```python
from build123d import *

# Parameters (mm, degrees)
CROQUIS1_R              = 10
SALIENTE_EXTRUIR1_DEPTH = 100
CROQUIS2_R              = 7.5
SALIENTE_EXTRUIR2_DEPTH = 15
CROQUIS3_R              = 5
SALIENTE_EXTRUIR3_DEPTH = 16
REDONDEO1_R             = 4
CHAFL_N1_SIZE           = 1.99
CHAFL_N1_SIZE2          = 0.496162726
CROQUIS4_W              = 3.793672416
CROQUIS4_H              = 8.169837842
SALIENTE_EXTRUIR4_DEPTH = 16
CHAFL_N2_SIZE           = 12
CHAFL_N2_SIZE2          = 6.38051318
REDONDEO2_R             = 10


with BuildPart() as part:
    # Croquis1 → Saliente-Extruir1 (new body)
    with BuildSketch(Plane(origin=(0, 0, 0), x_dir=(1, 0, 0), z_dir=(0, 1, 0))):
        with Locations(Location((0, 0, 0), (0, 0, 270))):
            Circle(CROQUIS1_R)
    extrude(amount=SALIENTE_EXTRUIR1_DEPTH)

    # Croquis2 → Saliente-Extruir2 (add)
    with BuildSketch(Plane.XZ):
        with Locations(Location((0, 0, 0), (0, 0, 270))):
            Circle(CROQUIS2_R)
    extrude(amount=SALIENTE_EXTRUIR2_DEPTH)

    # Croquis3 → Saliente-Extruir3 (add)
    with BuildSketch(Plane.XZ.offset(15)):
        with Locations(Location((0, 0, 0), (0, 0, 270))):
            Circle(CROQUIS3_R)
    extrude(amount=SALIENTE_EXTRUIR3_DEPTH)

    # Redondeo1
    # the kernel refuses this fillet: 4 mm, written as the material it takes off along each edge
    with BuildSketch(Plane(origin=(0, 0, 0), x_dir=(0, 0, 1), z_dir=(-1, 0, 0))) as redondeo1_piece_1:
        with BuildLine():
            CenterArc((6, 3.708099244), REDONDEO1_R, 292.024312837, 67.975687163)
            Line((7.5, 0), (7.53, -0.074161985))
            ThreePointArc((7.53, -0.074161985), (8.75, -0.08), (10, -0.08))
            Line((10, -0.08), (10.08, 0))
            Line((10.08, 0), (10.08, 3.708099244))
            Line((10.08, 3.708099244), (10, 3.708099244))
        make_face()
    revolve(axis=Axis((0, 0, 0), (0, 1, 0)), mode=Mode.SUBTRACT)

    # Chaflán1
    chafl_n1_edges = [part.edges().sort_by_distance(p)[0] for p in [
        (0, -31, 5),
    ]]
    chafl_n1_side = [part.faces().sort_by_distance(p)[0] for p in [
        (0, -23, 5),
    ]]
    chamfer(chafl_n1_edges, length=CHAFL_N1_SIZE, length2=CHAFL_N1_SIZE2, reference=chafl_n1_side[0])

    # Croquis4 → Saliente-Extruir4 (add)
    with BuildSketch(Plane.XZ.offset(31)):
        Rectangle(CROQUIS4_W, CROQUIS4_H)
    extrude(amount=SALIENTE_EXTRUIR4_DEPTH)

    # Chaflán2
    chafl_n2_edges = [part.edges().sort_by_distance(p)[0] for p in [
        (0, -47, -4.084918921),
    ]]
    chafl_n2_side = [part.faces().sort_by_distance(p)[0] for p in [
        (0, -39, -4.084918921),
    ]]
    chamfer(chafl_n2_edges, length=CHAFL_N2_SIZE, length2=CHAFL_N2_SIZE2, reference=chafl_n2_side[0])

    # Redondeo2
    redondeo2_edges = [part.edges().sort_by_distance(p)[0] for p in [
        (0, 100, -10),
    ]]
    fillet(redondeo2_edges, radius=REDONDEO2_R)


solid = part.part
```
The model under review builds one solid part; all positions refer to its coordinate system, in mm. A direction names the side the tool comes from. Give positions to 0.01 mm unless a question says otherwise; leave off trailing zeros. Write each loop counter-clockwise with the first axis right and the second up, starting at its lowest first coordinate (ties: lowest second). Pieces come first, ordered by that corner, then holes. Notation, with made-up numbers: M 9,87.25 L 21,87.25 A21 ccw 21,96.25 Z; hole C 58.5,20.25 d3. An arc over 180 degrees is marked long. Answer in a Markdown table with one row per item.
Item 1: Tool access review of faces 1 (the face through (0, -39, 4.085)), 2 (the face through (0, -33, -4.085)), 3 (the face through (-3, -31, 0)), 4 (the face through (-4.88, -21.91, 1.08)): name each direction out of +Z, -Z, +X, -X, +Y, -Y from which nothing blocks a thin tool from reaching the whole face with its end or side.
Check sheet entries:
| item | result |
|---|---|
| face 1 | +Z, +X, -X, -Y |
| face 2 | -Z, +X, -X, -Y |
| face 3 | +Z, -Z, -X, -Y |
| face 4 | -Y |
Item 2: Add section A-A on x = 0. Give the boundary of the cut face in (y, z).
Check sheet entries:
| item | result |
|---|---|
| outline | M -47,2.3 L -35,-4.08 L -31,-4.08 L -31,-4.5 L -29.01,-5 L -15,-5 L -15,-7.5 L 0,-7.5 A4 ccw 3.71,-10 L 90,-10 A10 ccw 90,10 L 3.71,10 A4 ccw 0,7.5 L -15,7.5 L -15,5 L -29.01,5 L -31,4.5 L -31,4.08 L -47,4.08 Z |
Item 3: Add section C-C on y = -19. Give the boundary of the cut face in (x, z), plus the area to 3 significant figures.
Check sheet entries:
| item | result |
|---|---|
| outline | C 0,0 d10 |
| area | 78.5 mm2 |
Item 4: For P1, Ø8, axis at x = 2.5, z = -8, coming from the -Y side; P2, Ø10, axis at x = 7.5, y = 32.5, coming from the -Z side; P3, Ø2, axis at x = -5, z = -6, coming from the -Y side, all flat-tipped, find the tip position at first contact; note any pin that passes through.
Check sheet entries:
| item | result |
|---|---|
| P1 | y = -35.07 |
| P2 | z = -9.68 |
| P3 | y = -15 |
Item 5: Add section D-D on y = 43. Give the boundary of the cut face in (x, z).
Check sheet entries:
| item | result |
|---|---|
| outline | C 0,0 d20 |
Item 6: Add section B-B on z = 0. Give the boundary of the cut face in (x, y), plus the area to 3 significant figures.
Check sheet entries:
| item | result |
|---|---|
| outline | M -10,3.71 A4 ccw -7.5,0 L -7.5,-15 L -5,-15 L -5,-29.01 L -4.5,-31 L -1.9,-31 L -1.9,-42.68 L 1.9,-42.68 L 1.9,-31 L 4.5,-31 L 5,-29.01 L 5,-15 L 7.5,-15 L 7.5,0 A4 ccw 10,3.71 L 10,90 A10 ccw -10,90 Z |
| area | 2,380 mm2 |
Item 7: For line 1 along Z through (x, y) = (-0.25, -11.5); line 2 along Z through (x, y) = (-0.25, -31.5); line 3 along X through (y, z) = (74, 0.25), list the stretches that pass through material, from the lowest coordinate up.
Check sheet entries:
| item | result |
|---|---|
| line 1 | -7.5 to 7.5 |
| line 2 | -4.08 to 4.08 |
| line 3 | -10 to 10 |
